Source: CAD feature listing. Evaluate the final solid. Frame: model axes, mm. Coordinates: 2 decimals unless noted, no trailing zeros.
```python
from build123d import *

# Parameters (mm, degrees)
SKETCH1_R           = 2
SKETCH1_R_2         = 1
BOSS_EXTRUDE1_DEPTH = 10


with BuildPart() as part:
    # Sketch1 → Boss-Extrude1 (new body)
    with BuildSketch(Plane(origin=(0, 0, 0), x_dir=(1, 0, 0), z_dir=(0, 1, 0))):
        with BuildLine():
            Line((-43.980681388, -35.900071191), (-49.199029144, -26.673592784))
            add(Edge.make_bspline(
                [(-49.199029144, -26.673592784), (-31.845281334, -4.900517613), (-24.966664763, -2.13955382), (-5.316002055, 8.469954082)],
                knots=[0, 0, 0, 0, 1, 1, 1, 1], degree=3))
            ThreePointArc((-5.316002055, 8.469954082), (8.469954082, 5.316002055), (5.316002055, -8.469954082))
            add(Edge.make_bspline(
                [(-43.980681388, -35.900071191), (-21.812551229, -8.740215805), (-12.045610471, -15.281217208), (5.316002055, -8.469954082)],
                knots=[0, 0, 0, 0, 1, 1, 1, 1], degree=3))
        make_face()
        Circle(SKETCH1_R, mode=Mode.SUBTRACT)
        with Locations((-20.788744537, -8.469954082)):
            Circle(SKETCH1_R_2, mode=Mode.SUBTRACT)
    extrude(amount=BOSS_EXTRUDE1_DEPTH)


solid = part.part
```
1. Ray query, line 1 (Z direction, x = 0, y = 5.75); line 2 (Z direction, x = -1, y = 5.25); line 3 (X direction, y = 3, z = 0). Return the intervals inside material, ascending.
Findings:
line 1: z = -10 to -2, 2 to 10.25
line 2: z = -9.95 to -1.73, 1.73 to 10.52
line 3: x = -20.71 to -2, 2 to 10
2. Section query A-A on y = 6. Count the separate pieces of the cut face and the enclosed holes in it, plus the area to 3 significant figures.
Findings:
separate pieces: 1
enclosed holes: 2
area: 920 mm2
3. Pin query (flat end, axial travel): P1, Ø6, axis at x = 2, y = 4.5, coming from the +Z side; P2, Ø1.5, axis at x = 1.5, y = 4, coming from the +Z side; P3, Ø1.5, axis at x = 2.5, y = 2.5, coming from the -Z side. Return the tip coordinate at first contact, or that it passes through.
Findings:
P1: stops at z = 10.52
P2: stops at z = 10.03
P3: stops at z = -9.85
